from build123d import *

# Parameters (mm, degrees)
F0_W      = 59
F0_H      = 54
F1_DEPTH  = 5
F2_W      = 42
F2_H      = 42
F3_DEPTH  = 9.75
F5_DEPTH  = 33
F6_R      = 1.6
F6_R_2    = 11.5
F7_DEPTH  = 14.751
F8_SIZE   = 3
F9_R      = 1.6
F10_DEPTH = 2.5
F12_DEPTH = 10.6937211186
F14_DEPTH = 5.001
F16_DEPTH = 20
F18_DEPTH = 20
F19_R     = 2
F20_W     = 5.6
F20_H     = 20
F20_H_2   = 5
F20_W_2   = 5
F20_H_3   = 5.6
F20_W_3   = 20
F21_DEPTH = 3
F22_SIZE  = 2.99999
F23_R     = 1.9824364908
F23_R_2   = 2.1
F24_DEPTH = 5.001


# Not quite as in the source:
# - a fillet or chamfer is up to 0.001 mm smaller than in the source, because OpenCascade refuses the exact size


with BuildPart() as f1:
    # F0 (on Top) → F1 (new body)
    with BuildSketch(Plane.XY):
        with Locations((29.5, 27)):
            Rectangle(F0_W, F0_H)
    extrude(amount=F1_DEPTH)

    # F2 (on face) → F3 (join)
    with BuildSketch(Plane.XY.offset(5)):
        with Locations((38, 21)):
            Rectangle(F2_W, F2_H)
    extrude(amount=F3_DEPTH)

    # F4 (on face) → F5 (cut)
    with BuildSketch(Plane.YZ.offset(59)):
        Polygon((0, 6.5), (0, 0), (33, 0), (19, 6.5), align=None)
    extrude(amount=-F5_DEPTH, mode=Mode.SUBTRACT)

    # F6 (on face) → F7 (cut, through all)
    with BuildSketch(Plane.XY.offset(14.75)):
        with Locations((22.8, 36.2)):
            Circle(F6_R)
        with Locations((38, 21)):
            Circle(F6_R_2)
        with Locations((53.2, 36.2)):
            Circle(F6_R)
        with Locations((22.8, 5.8)):
            Circle(F6_R)
        with Locations((53.2, 5.8)):
            Circle(F6_R)
        with Locations((29.8, 5.8)):
            Circle(F6_R)
    extrude(amount=-F7_DEPTH, mode=Mode.SUBTRACT)

    # F8
    f8_edges = [f1.edges().sort_by_distance(p)[0] for p in [
        (59, 42, 9.875),
        (59, 0, 10.625),
    ]]
    chamfer(f8_edges, length=F8_SIZE)

    # F9 (on face) → F10 (cut)
    with BuildSketch(Plane.XY.offset(14.75)):
        Polygon((31.417729554, 3.0006632601), (33.0331615075, 5.8013265202), (31.4154319535, 8.6006632601), (28.182270446, 8.5993367399), (26.5668384925, 5.7986734798), (28.1845680465, 2.9993367399), align=None)
        with Locations((29.8, 5.8)):
            Circle(F9_R, mode=Mode.SUBTRACT)
    extrude(amount=-F10_DEPTH, mode=Mode.SUBTRACT)

    # F11 (on face) → F12 (cut, through all)
    with BuildSketch(Plane.XZ):
        with BuildLine():
            Line((32.9, 9.5), (32.9, 6.5))
            Line((32.9, 6.5), (41.1, 6.5))
            Line((41.1, 6.5), (41.1, 9.5))
            ThreePointArc((41.1, 9.5), (37, 13.6), (32.9, 9.5))
        make_face()
    extrude(amount=-F12_DEPTH, mode=Mode.SUBTRACT)

    # F13 (on face) → F14 (cut, through all)
    with BuildSketch(Plane.XY.offset(5)):
        Polygon((17, 42), (56, 42), (59, 42), (59, 54), (0, 54), (0, 0), (17, 0), align=None)
    extrude(amount=-F14_DEPTH, mode=Mode.SUBTRACT)

    # F15 (on face) → F16 (join)
    with BuildSketch(Plane(origin=(0, 42, 0), x_dir=(-1, 0, 0), z_dir=(0, 1, 0))):
        Polygon((-56, 5), (-59, 5), (-59, 0), (-17, 0), (-17, 5), align=None)
    extrude(amount=F16_DEPTH)

    # F17 (on face) → F18 (join)
    with BuildSketch(Plane(origin=(17, 0, 0), x_dir=(0, -1, 0), z_dir=(-1, 0, 0))):
        Polygon((-42, 5), (-62, 5), (-62, 0), (0, 0), (0, 5), align=None)
    extrude(amount=F18_DEPTH)

    # F19
    f19_edges = [f1.edges().sort_by_distance(p)[0] for p in [
        (-3, 62, 2.5),
        (-3, 31, 0),
        (28, 62, 0),
    ]]
    fillet(f19_edges, radius=F19_R)

    # F20 (on face) → F21 (join)
    with BuildSketch(Plane.XY.offset(5)):
        with Locations((7, 21)):
            Rectangle(F20_W, F20_H)
        with Locations((7, 39.5)):
            Rectangle(F20_W, F20_H_2)
        with Locations((7, 2.5)):
            Rectangle(F20_W, F20_H_2)
        with Locations((19.5, 52)):
            Rectangle(F20_W_2, F20_H_3)
        with Locations((38, 52)):
            Rectangle(F20_W_3, F20_H_3)
        with Locations((56.5, 52)):
            Rectangle(F20_W_2, F20_H_3)
    extrude(amount=F21_DEPTH)

    # F22 (size 3 in the source; OpenCascade refuses exactly that, so slightly less here)
    f22_edges = [f1.edges().sort_by_distance(p)[0] for p in [
        (54, 52, 8),
        (48, 52, 8),
        (28, 52, 8),
        (22, 52, 8),
        (7, 37, 8),
        (7, 31, 8),
        (7, 11, 8),
        (7, 5, 8),
    ]]
    chamfer(f22_edges, length=F22_SIZE)

    # F23 (on face) → F24 (cut, through all)
    with BuildSketch(Plane.XY.offset(5)):
        with Locations((7, 8)):
            Circle(F23_R)
        with Locations((7, 34)):
            Circle(F23_R_2)
        with Locations((25, 52)):
            Circle(F23_R_2)
        with Locations((51, 52)):
            Circle(F23_R_2)
    extrude(amount=-F24_DEPTH, mode=Mode.SUBTRACT)


solid = f1.part
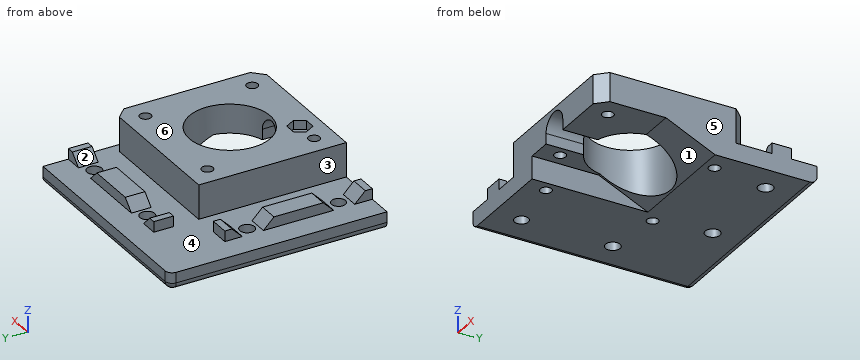
Source: CAD feature listing. Evaluate the final solid. Frame: model axes, mm. Face numbers are marked on the shaded views. A direction names the side the tool comes from. Give positions to 0.01 mm unless a question says otherwise; leave off trailing zeros. Write each loop counter-clockwise with the first axis right and the second up, starting at its lowest first coordinate (ties: lowest second). Pieces come first, ordered by that corner, then holes. Notation, with made-up numbers: (65, -5) - (78, -5) arc R15 ccw to (78, 1) - close; hole circle Ø8 at (27, 44.25). An arc over 180 degrees is marked (long way). Write item = value, one per line. Start each with the question number.
Q1. Draft query along X for the marked faces 4, 5 and 6. Return one class per face: +X half, -X half, draft (parallel to the pull), parting line (faces both ways), or undercut.
Q2. Pin query (flat end, axial travel): pin 1 Ø5 at (x, y) = (45.5, 24) entering from +Z; pin 2 Ø6 at (x, z) = (16, 11) entering from +Y; pin 3 Ø9 at (x, y) = (53, 5.5) entering from -Z; pin 4 Ø5.5 at (x, y) = (51, 52) entering from +Z. Return the tip coordinate at first contact, or that it passes through.
Q3. Cut plane A-A, the plane y = 52. Give the number of separate pieces and of enclosed holes in the cut face, then the cut area to 3 significant figures.
Q4. Reachability of the marked faces 1, 2 and 3 from +Z, -Z, +X, -X, +Y, -Y: full face, straight path, thin tool, end or side. Return the list, or none.
Q5. Cut plane D-D, the plane y = 24.5. Return loops of the section in (x, z).
Q6. Material intervals for probe 1 along Y at (x, z) = (22.8, 9); probe 2 along Y at (x, z) = (29.8, 10.2); probe 3 along Y at (x, z) = (50.5, 8.5), sorted ascending.
Q7. Cut plane C-C, the plane x = 43. Return loops of the section in (y, z), then the cut area to 3 significant figures.
Computed values:
q1.face_4 = undercut
q1.face_5 = +X half
q1.face_6 = draft
q2.pin_1 = through
q2.pin_2 = 42
q2.pin_3 = 6.5
q2.pin_4 = 5
q3.separate_pieces = 3
q3.enclosed_holes = 0
q3.area = 339 mm²
q4.face_1 = -Z, +X, -Y
q4.face_2 = +Z, +Y
q4.face_3 = +Z, +Y, -Y
q5.outline = (-3, 2) arc R2 ccw to (-1, 0) - (26, 0) - (26, 3.95) - (27.05, 3.95) - (27.05, 14.75) - (17, 14.75) - (17, 5) - (9.8, 5) - (9.8, 8) - (4.2, 8) - (4.2, 5) - (-3, 5) - close; (48.95, 3.95) - (59, 3.95) - (59, 14.75) - (48.95, 14.75) - close
q6.probe_1 = 0 to 4.2, 7.4 to 34.6, 37.8 to 42
q6.probe_2 = 0 to 4.2, 7.4 to 12.94, 29.06 to 42
q6.probe_3 = 0 to 42
q7.outline = (0, 6.5) - (10.64, 6.5) - (10.64, 14.75) - (0, 14.75) - close; (31.36, 0.76) - (33, 0) - (60, 0) arc R2 ccw to (62, 2) - (62, 5) - (54.8, 5) - (54.8, 8) - (49.2, 8) - (49.2, 5) - (42, 5) - (42, 14.75) - (31.36, 14.75) - close
q7.area = 360 mm²
